Autodesk Inventor part; units mm, degrees
ref_plane "YZ Plane" through (0, 0, 0) normal (1, 0, 0) x (0, 1, 0)
ref_plane "XZ Plane" through (0, 0, 0) normal (0, 1, 0) x (-1, 0, 0)
ref_plane "XY Plane" through (0, 0, 0) normal (0, 0, 1) x (1, 0, 0)
sketch "Sketch1" plane through (0, 0, 0) normal (0, 1, 0) x (-1, 0, 0)
  circle A0 centre (0, 0) radius 6.35
  dimension "d0" = 12.7
extrude "Extrusion1" add sketch "Sketch1" along normal blind 12.7
sketch "Sketch2" plane through (0, 0, 0) normal (0, 0, 1) x (1, 0, 0)
  circle A0 centre (0, 60.325) radius 57.15
  line L0 (-41.9347, 3.175) -> (51.5907, 3.175) construction
  point P0 (0, 0)
  dimension "d3" = 114.3
  dimension "d4" = 3.175
extrude "Extrusion2" cut sketch "Sketch2" along normal through all both and the other way through all
sketch "Sketch4" plane through (0, 0, 0) normal (0, -1, 0) x (1, 0, 0)
  point P0 (0, 0)
  point P1 (0, 0)
hole "Hole1" at (0, 0, 0) direction (0, 1, 0) diameter 6.7564 end through all
properties part number "Spacers" material "Aluminum 6061"
Here's how the part is built. I have some questions about the finished solid (model axes, mm). Coordinates: 2 decimals unless noted, no trailing zeros. Order: outer loops, then holes, each group sorted by start corner. A loop starts at its lowest first (then second) coordinate and runs counter-clockwise, first axis right, second up. Notation, with made-up numbers: M 60,53 L 71,53 A29 cw 71,80 Z; hole C 32.25,48 d4. An arc over 180 degrees is marked long. Answer as a JSON object with one key per item and string values. Group by question number.
(1) Suppose I cut it at B-B, the plane x = 0. Please give me the cut outline in (y, z) (3 decimals).
(2) If we mould it in two halves opening along X, with no side actions, what happens to faces 1 (the face through (2.056, 1.66, 2.681)), 2 (the face through (6.344, 1.74, -0.279)), 3 (the face through (-3, 0, -3))? For each: released by +X, released by -X, zero draft, split by the parting line, or undercut.
(3) Suppose I cut it at C-C, the plane y = 0.55. Please give me the cut outline in (x, z), then the cut area to 3 significant figures.
(4) I need wall thicknesses on probe 1 along X at (y, z) = (1, 0); probe 2 along Z at (x, y) = (2.5, 0.6). Which ranges of each line are inside material? Lowest first, please.
(5) For pin 1 (4 mm diameter, centred on x = 0, z = 0, fed in from -Y); pin 2 (2 mm diameter, centred on x = 4, z = -1.5, fed in from +Y), each with a flat end and sliding along its axis, tell me the tip position at first contact or that it passes through.
(6) Suppose I cut it at D-D, the plane x = 5. Please give me the cut outline in (y, z).
(7) Suppose I cut it at A-A, the plane z = 0. Please give me the cut outline in (x, y) (3 decimals).
Values found:
{
 "1": {"outline": "M 0,-6.35 L 3.175,-6.35 L 3.175,-3.378 L 0,-3.378 Z; M 0,3.378 L 3.175,3.378 L 3.175,6.35 L 0,6.35 Z"},
 "2": {"face 1": "undercut", "face 2": "split by the parting line", "face 3": "zero draft"},
 "3": {"outline": "C 0,0 d12.7; hole C 0,0 d6.76", "area": "90.8 mm^2"},
 "4": {"probe 1": "x = -6.35 to -3.38, 3.38 to 6.35", "probe 2": "z = -5.84 to -2.27, 2.27 to 5.84"},
 "5": {"pin 1": "passes through", "pin 2": "stops at y = 3.39"},
 "6": {"outline": "M 0,-3.91 L 3.39,-3.91 L 3.39,3.91 L 0,3.91 Z"},
 "7": {"outline": "M -6.35,0 L -3.378,0 L -3.378,3.275 A57.15 cw -6.35,3.529 Z; M 3.378,0 L 6.35,0 L 6.35,3.529 A57.15 cw 3.378,3.275 Z"}
}
